Part print with two shaded views. Sizes in mm from the minimum x, y, z corner. Coordinates: 2 decimals unless noted, no trailing zeros. Loops run counter-clockwise (first coordinate to the right, second up) from the corner with the lowest first, then second, coordinate; pieces in that order, holes last. Notation, with made-up numbers: (-21, -11.75) -> (7, -11.75) arc R17 cw to (7, 20.25) -> close; hole circle Ø5 at (81.25, -18). An arc over 180 degrees is marked (long way). Use one line per item in the form item = value.
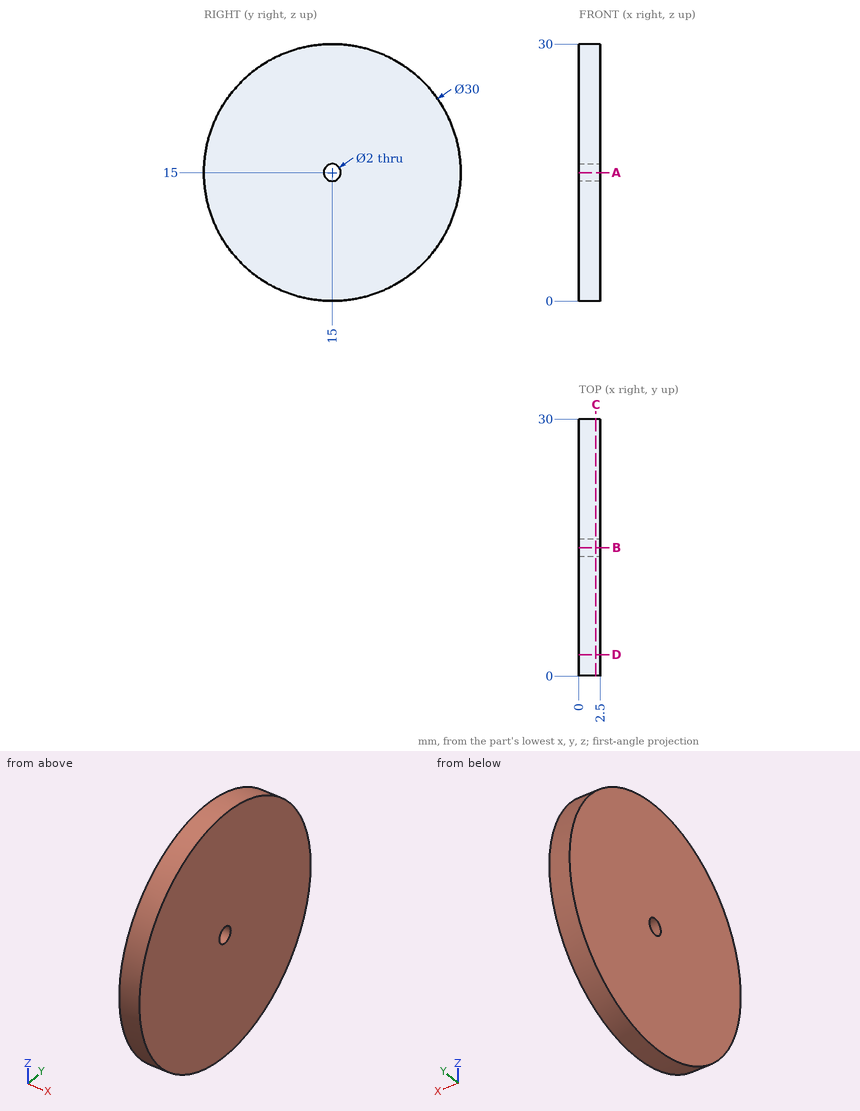
Q1. Pin check, flat tips, straight feed: pin 1 Ø1.5 at (x, y) = (0.5, 22.5) entering from +Z; pin 2 Ø1.6 at (y, z) = (15, 15) entering from +X; pin 3 Ø1.5 at (x, y) = (1.5, 24) entering from +Z. Stop position of each tip, or through.
Result:
pin_1 = 28.4
pin_2 = through
pin_3 = 27.53
Q2. Band-saw the part on C-C, the plane x = 2. Write the cut outline in (y, z).
Result:
outline = circle Ø30 at (15, 15); hole circle Ø2 at (15, 15)
Q3. Wall check: line 1 along Y through (x, z) = (2.2, 5); line 2 along Z through (x, y) = (0.2, 9); line 3 along Y through (x, z) = (0.5, 3). Give the ranges that are in metal, low to high.
Result:
line_1 = 3.82 to 26.18
line_2 = 1.25 to 28.75
line_3 = 6 to 24
Q4. Band-saw the part on D-D, the plane y = 2.5. Write the cut outline in (x, z).
Result:
outline = (0, 6.71) -> (2.5, 6.71) -> (2.5, 23.29) -> (0, 23.29) -> close
Q5. Band-saw the part on A-A, the plane z = 15. Write the cut outline in (x, y), and give its area (3 significant figures).
Result:
outline = (0, 0) -> (2.5, 0) -> (2.5, 14) -> (0, 14) -> close; (0, 16) -> (2.5, 16) -> (2.5, 30) -> (0, 30) -> close
area = 70.0 mm2
